The drawing under review shows one solid part. Ordinate dimensions are in mm from its lowest x, y, z. Give positions to 0.01 mm unless a question says otherwise; leave off trailing zeros. Order: outer loops, then holes, each group sorted by start corner. A loop starts at its lowest first (then second) coordinate and runs counter-clockwise, first axis right, second up. Notation, with made-up numbers: (-1.5, 26) - (25.5, 26) arc R23 cw to (25.5, 51) - close; hole circle Ø2 at (48.5, -38). An arc over 180 degrees is marked (long way). Use CSV: the item, a comma, the result in double quotes. Start each with the question number.
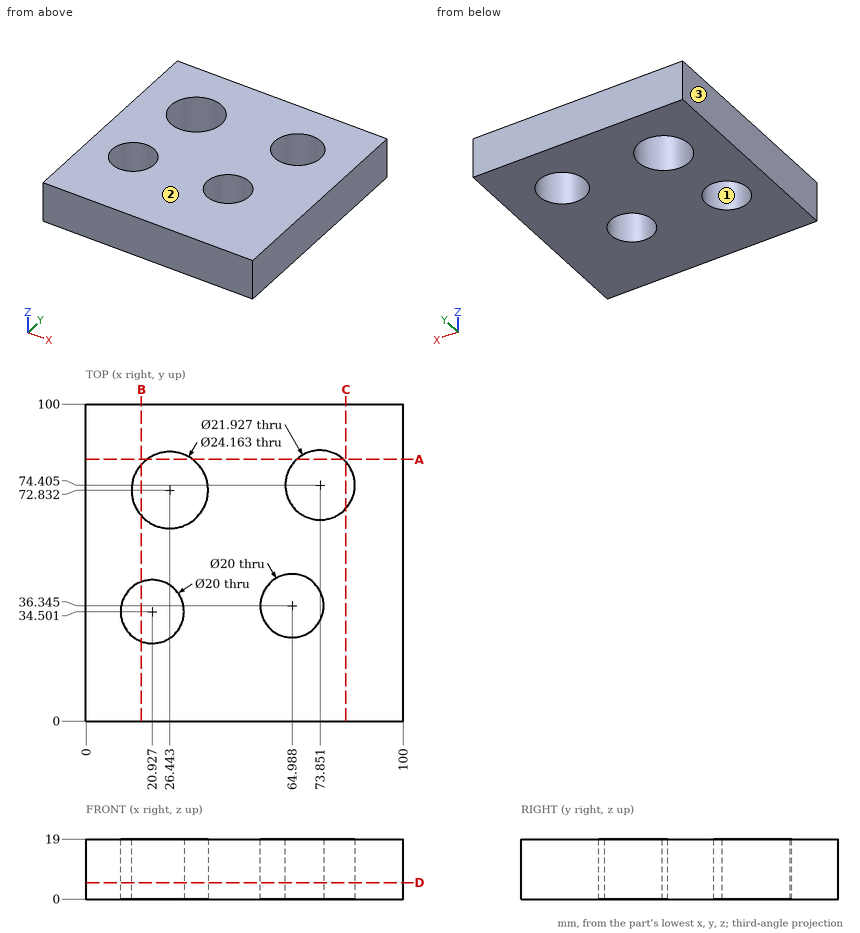
1. To check wall thickness, follow L1, parallel to X at y = 36, z = 12.25 (1 decimal); L2, parallel to X at y = 74, z = 13 (1 decimal); L3, parallel to Y at x = 56, z = 2.5 (1 decimal). State the ranges of each line that lie inside material, in increasing order. Write a range as [from, to].
2. Mouldability with a two-part tool opening along X and no side actions: class the marked faces 1, 2 and 3 as pulls with the +X half, pulls with the -X half, needs draft (parallel to the pull), parting line crosses it, or undercut.
3. Consider section C-C (x = 82). Give the boundary of the cut face in (y, z).
4. Consider section D-D (z = 5.25). State how many separate pieces and enclosed holes the cut face has.
5. Consider section B-B (x = 17.5). Give the boundary of the cut face in (y, z) (1 decimal), and give its area (3 significant figures).
6. Consider section A-A (y = 82.5). Give the boundary of the cut face in (x, z), and give its area (3 significant figures).
Answers follow:
1,L1,"x = [0, 11], [30.8, 55], [75, 100]"
1,L2,"x = [0, 14.4], [38.5, 62.9], [84.8, 100]"
1,L3,"y = [0, 32], [40.7, 100]"
2,face 1,"undercut"
2,face 2,"needs draft"
2,face 3,"pulls with the -X half"
3,outline,"(0, 0) - (67.07, 0) - (67.07, 19) - (0, 19) - close; (81.74, 0) - (100, 0) - (100, 19) - (81.74, 19) - close"
4,separate pieces,"1"
4,enclosed holes,"4"
5,outline,"(0, 0) - (25.1, 0) - (25.1, 19) - (0, 19) - close; (43.9, 0) - (64.7, 0) - (64.7, 19) - (43.9, 19) - close; (81, 0) - (100, 0) - (100, 19) - (81, 19) - close"
5,area,"1,230 mm^2"
6,outline,"(0, 0) - (19.2, 0) - (19.2, 19) - (0, 19) - close; (33.69, 0) - (66.46, 0) - (66.46, 19) - (33.69, 19) - close; (81.24, 0) - (100, 0) - (100, 19) - (81.24, 19) - close"
6,area,"1,340 mm^2"
